Here's how the part is built. I have some questions about the finished solid (model axes, mm). A direction names the side the tool comes from. Give positions to 0.01 mm unless a question says otherwise; leave off trailing zeros. Write each loop counter-clockwise with the first axis right and the second up, starting at its lowest first coordinate (ties: lowest second). Pieces come first, ordered by that corner, then holes. Notation, with made-up numbers: M 51,54 L 105,54 A21 ccw 105,59 Z; hole C 33.5,31.25 d3. An arc over 180 degrees is marked long. Answer as CSV lines item,"result". Start each with the question number.
Q1. Thinking about a two-plate mould opening in Y: for faces 1 (the flat face through (0, 9.525, 0)), 2 (the flat face through (4.365, 0, 0)), 3 (the conical face through (1.955, -2.27, -0.156)), 4 (the cylindrical face through (-1.781, -3.495, -0.563)), which applies, +Y half, -Y half, draft (parallel to the pull), parting line (faces both ways), or undercut?
Q2. For pin 1 (1 mm diameter, centred on y = -7.5, z = 1.5, fed in from +X), with a flat end and sliding along its axis, tell me the tip position at first contact or that it passes through.
Q3. Suppose I cut it at A-A (x = -0.25). Write out the boundary of the cut face in (y, z) (3 decimals).
Q4. On a 3-axis mill with a long thin cutter (end or side, diameter ignored), from which of +Z, -Z, +X, -X, +Y, -Y can I reach the whole of each face in a straight line? I mean faces 5 (the flat face through (0, -9.525, 0)), 6 (the cylindrical face through (3.148, 6.306, 0.366)). Say none if no direction works.
Q5. If I drill on line 1 along Y through (x, z) = (-4.5, 0) (3 decimals); line 2 along X through (y, z) = (6.75, 0) (3 decimals); line 3 along Y through (x, z) = (-2.75, -0.75) (3 decimals), over which ranges is the centre line in solid material (lowest first)?
```python
from build123d import *

# Parameters (mm, degrees)
SKETCH1_W                 = 10
SKETCH1_H                 = 19.05
BOSS_EXTRUDE1_DEPTH       = 3.175
F_2_CLEARANCE_HOLE1_D     = 2.4384
F_2_CLEARANCE_HOLE1_DEPTH = 6.35
F_2_CLEARANCE_HOLE1_TIP   = 0.732569267
F_2_CLEARANCE_HOLE2_D     = 2.4384
F_2_CLEARANCE_HOLE2_DEPTH = 6.35
F_2_CLEARANCE_HOLE2_TIP   = 0.732569267
FILLET1_R                 = 1.5875
SKETCH7_W                 = 0.635
SKETCH7_H                 = 6.35
CUT_EXTRUDE1_DEPTH        = 20.05
FILLET2_R                 = 2.54


with BuildPart() as part:
    # Sketch1 → Boss-Extrude1 (new body, symmetric)
    with BuildSketch(Plane.XY):
        Rectangle(SKETCH1_W, SKETCH1_H)
    extrude(amount=BOSS_EXTRUDE1_DEPTH, both=True)

    # #2 Clearance Hole1
    with Locations(Plane(origin=(0, 9.525, 0), x_dir=(-1, 0, 0), z_dir=(0, 1, 0))):
        with Locations((-1.985, 0)):
            Hole(F_2_CLEARANCE_HOLE1_D / 2, depth=F_2_CLEARANCE_HOLE1_DEPTH)
            with Locations((0, 0, -(F_2_CLEARANCE_HOLE1_DEPTH + F_2_CLEARANCE_HOLE1_TIP / 2))):  # 118° drill point
                Cone(0, F_2_CLEARANCE_HOLE1_D / 2, F_2_CLEARANCE_HOLE1_TIP, mode=Mode.SUBTRACT)

    # #2 Clearance Hole2
    with Locations(Plane.ZY.offset(5)):
        with Locations((0, -2.413)):
            Hole(F_2_CLEARANCE_HOLE2_D / 2, depth=F_2_CLEARANCE_HOLE2_DEPTH)
            with Locations((0, 0, -(F_2_CLEARANCE_HOLE2_DEPTH + F_2_CLEARANCE_HOLE2_TIP / 2))):  # 118° drill point
                Cone(0, F_2_CLEARANCE_HOLE2_D / 2, F_2_CLEARANCE_HOLE2_TIP, mode=Mode.SUBTRACT)

    # Fillet1
    fillet1_edges = [part.edges().sort_by_distance(p)[0] for p in [
        (5, 0, 3.175),
        (5, 0, -3.175),
    ]]
    fillet(fillet1_edges, radius=FILLET1_R)

    # Sketch7 → Cut-Extrude1 (cut, through all)
    with BuildSketch(Plane.XZ.offset(9.525)):
        with Locations((4.6825, 0)):
            Rectangle(SKETCH7_W, SKETCH7_H)
    extrude(amount=-CUT_EXTRUDE1_DEPTH, mode=Mode.SUBTRACT)

    # Fillet2
    fillet2_edges = [part.edges().sort_by_distance(p)[0] for p in [
        (4.365, 0, -2.8575),
        (4.365, 0, 2.8575),
    ]]
    fillet(fillet2_edges, radius=FILLET2_R)


solid = part.part
```
Resolved:
1,face 1,"+Y half"
1,face 2,"draft"
1,face 3,"undercut"
1,face 4,"undercut"
2,pin 1,"x = 4.34"
3,outline,"M -9.525,-3.175 L 9.525,-3.175 L 9.525,3.175 L -9.525,3.175 Z; hole C -2.413,0 d2.438"
4,face 5,"+Z, -Z, +X, -X, -Y"
4,face 6,"+Y"
5,line 1,"-9.525 to -3.632, -1.194 to 9.525"
5,line 2,"-5 to 0.766, 3.204 to 4.365"
5,line 3,"-9.525 to -3.374, -1.452 to 9.525"
